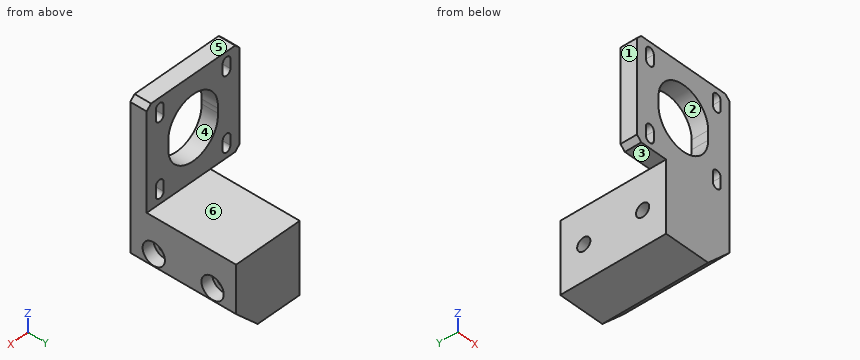
Autodesk Inventor part; units mm, degrees
ref_plane "YZ Plane" through (0, 0, 0) normal (1, 0, 0) x (0, 1, 0)
ref_plane "XZ Plane" through (0, 0, 0) normal (0, 1, 0) x (-1, 0, 0)
ref_plane "XY Plane" through (0, 0, 0) normal (0, 0, 1) x (1, 0, 0)
sketch "Sketch1" plane through (0, 0, 0) normal (0, 1, 0) x (-1, 0, 0)
  line L0 (-21.5, 21.5) -> (21.5, 21.5)
  line L1 (21.5, 21.5) -> (21.5, -21.5)
  line L2 (21.5, -21.5) -> (-21.5, -21.5)
  line L3 (-21.5, -21.5) -> (-21.5, 21.5)
  line L4 (-21.5, 21.5) -> (21.5, -21.5) construction
  line L5 (21.5, 21.5) -> (-21.5, -21.5) construction
  circle A0 centre (0, 0) radius 11.5
  circle A1 centre (15.5, 15.5) radius 1.8
  circle A2 centre (-15.5, 15.5) radius 1.8
  circle A3 centre (-15.5, -15.5) radius 1.8
  circle A4 centre (15.5, -15.5) radius 1.8
  dimension "d0" = 23
  dimension "d1" = 43
  dimension "d2" = 43
  dimension "d3" = 3.6
  dimension "d5" = 31
  dimension "d6" = 31
extrude "Extrusion1" add sketch "Sketch1" along normal blind 7
sketch "Sketch6" plane through (0, 0, 0) normal (0, -1, 0) x (1, 0, 0)
  line L0 (21.5, -21.5) -> (-21.5, -21.5)
  line L1 (-8, -21.5) -> (-8, -51.5)
  line L2 (21.5, -21.5) -> (-8, -21.5)
  line L3 (-8, -21.5) -> (-8, -51.5)
  line L4 (-8, -51.5) -> (21.5, -51.5)
  line L5 (21.5, -51.5) -> (21.5, -21.5)
  point P0 (0, 0)
  dimension "d26" = 8
  dimension "d27" = 30
extrude "Extrusion5" add sketch "Sketch6" against normal blind 45
chamfer "Chamfer1" distance 2 angle 45 3 edges at (21.5, 3.5, 21.5) (-21.5, 3.5, 21.5) (-21.5, 3.5, -21.5)
sketch "Sketch7" plane through (21.5, 0, -51.5) normal (1, 0, 0) x (0, 0, -1)
  circle A0 centre (-15, 35) radius 2.8
  circle A1 centre (-15, 10) radius 2.8
  line L0 (0, 0) -> (0, 45)
  line L1 (-71, 7) -> (-30, 7)
  line L2 (-71, 0) -> (0, 0)
  line L3 (-30, 45) -> (0, 45)
  point P0 (-51.5, 0)
  dimension "d33" = 5.6
  dimension "d34" = 5.6
  dimension "d35" = 15
  dimension "d37" = 10
  dimension "d38" = 10
extrude "Extrusion6" cut sketch "Sketch7" against normal through all
sketch "Sketch8" plane through (21.5, 0, -51.5) normal (1, 0, 0) x (0, 0, -1)
  circle A0 centre (-15, 35) radius 2.8
  circle A1 centre (-15, 35) radius 4.75
  circle A2 centre (-15, 10) radius 2.8
  circle A3 centre (-15, 10) radius 4.75
  point P0 (-51.5, 0)
  dimension "d41" = 9.5
  dimension "d42" = 9.5
extrude "Extrusion7" cut sketch "Sketch8" against normal blind 5 contours A0 | A1 | A2 | A3
chamfer "Chamfer2" distance 10 angle 45 1 edges at (21.5, 22.5, -51.5)
sketch "Sketch9" plane through (0, 0, 0) normal (0, -1, 0) x (1, 0, 0)
  line L0 (13.7, 17.5) -> (17.3, 17.5)
  line L1 (17.3, 17.5) -> (17.3, 13.5)
  line L2 (17.3, 13.5) -> (13.7, 13.5)
  line L3 (13.7, 13.5) -> (13.7, 17.5)
  circle A0 centre (15.5, 15.5) radius 1.8
  line L4 (13.7, 17.5) -> (17.3, 13.5) construction
  line L5 (17.3, 17.5) -> (13.7, 13.5) construction
  line L6 (13.7, -13.5) -> (17.3, -13.5)
  line L7 (17.3, -13.5) -> (17.3, -17.5)
  line L8 (17.3, -17.5) -> (13.7, -17.5)
  line L9 (13.7, -17.5) -> (13.7, -13.5)
  circle A1 centre (15.5, -15.5) radius 1.8
  line L10 (13.7, -13.5) -> (17.3, -17.5) construction
  line L11 (17.3, -13.5) -> (13.7, -17.5) construction
  line L12 (-17.3, 17.5) -> (-13.7, 17.5)
  line L13 (-13.7, 17.5) -> (-13.7, 13.5)
  line L14 (-13.7, 13.5) -> (-17.3, 13.5)
  line L15 (-17.3, 13.5) -> (-17.3, 17.5)
  circle A2 centre (-15.5, 15.5) radius 1.8
  line L16 (-17.3, 17.5) -> (-13.7, 13.5) construction
  line L17 (-13.7, 17.5) -> (-17.3, 13.5) construction
  line L18 (-17.3, -13.5) -> (-13.7, -13.5)
  line L19 (-13.7, -13.5) -> (-13.7, -17.5)
  line L20 (-13.7, -17.5) -> (-17.3, -17.5)
  line L21 (-17.3, -17.5) -> (-17.3, -13.5)
  circle A3 centre (-15.5, -15.5) radius 1.8
  line L22 (-17.3, -13.5) -> (-13.7, -17.5) construction
  line L23 (-13.7, -13.5) -> (-17.3, -17.5) construction
  circle A4 centre (15.5, 17.5) radius 1.8
  circle A5 centre (15.5, -17.5) radius 1.8
  circle A6 centre (15.5, -13.5) radius 1.8
  circle A7 centre (-15.5, -17.5) radius 1.8
  circle A8 centre (-15.5, -13.5) radius 1.8
  circle A9 centre (-15.5, 13.5) radius 1.8
  circle A10 centre (-15.5, 17.5) radius 1.8
  circle A11 centre (15.5, 13.5) radius 1.8
  point P0 (0, 0)
  point P1 (-17.3, 17.5)
  point P2 (13.7, 17.5)
  point P3 (17.3, 13.5)
  dimension "d48" = 4
  dimension "d49" = 4
extrude "Extrusion8" cut sketch "Sketch9" against normal blind 10
sketch "Sketch10" plane through (0, 0, 0) normal (0, -1, 0) x (1, 0, 0)
  line L0 (-11.5, 2) -> (11.5, 2)
  line L1 (11.5, 2) -> (11.5, -2)
  line L2 (11.5, -2) -> (-11.5, -2)
  line L3 (-11.5, -2) -> (-11.5, 2)
  line L4 (-11.5, 2) -> (11.5, -2) construction
  line L5 (11.5, 2) -> (-11.5, -2) construction
  circle A0 centre (0, -2) radius 11.5
  circle A1 centre (0, 2) radius 11.5
  circle A2 centre (0, 0) radius 11.5
  point P0 (11.3248, 2)
  point P1 (-11.3248, 2)
  point P2 (-11.3248, -2)
  point P3 (11.3248, -2)
  point P4 (-11.5, 0)
  point P5 (11.5, 0)
  dimension "d52" = 4
extrude "Extrusion9" cut sketch "Sketch10" against normal blind 10
sketch "Sketch4" plane through (21.5, 0, 21.5) normal (1, 0, 0) x (0, 0, -1)
  line L0 (43, 45) -> (73, 45)
  line L1 (73, 45) -> (73, 0)
  line L2 (73, 0) -> (43, 0)
  line L3 (43, 0) -> (43, 45)
  line L4 (0, 0) -> (43, 0)
  line L5 (43, 0) -> (43, 7)
  point P0 (21.5, 0)
  dimension "d17" = 30
  dimension "d18" = 45
sketch "Sketch5" plane through (21.5, 0, 21.5) normal (1, 0, 0) x (0, 0, -1)
  circle A0 centre (58, 33) radius 2.75
  circle A1 centre (58, 12) radius 2.75
  line L0 (73, 45) -> (43, 45)
  line L1 (0, 0) -> (73, 0)
  point P0 (21.5, 0)
  dimension "d21" = 12
  dimension "d22" = 12
  dimension "d23" = 5.5
properties part number "ymotorholder"
Input: part model. Units: mm. Frame: model coordinates. Face numbers are marked on the shaded views. A direction names the side the tool comes from. Give positions to 0.01 mm unless a question says otherwise; leave off trailing zeros. Order: outer loops, then holes, each group sorted by start corner. A loop starts at its lowest first (then second) coordinate and runs counter-clockwise, first axis right, second up.
1. Set-up query: the marked faces 4, 5 and 6. Return all of +Z, -Z, +X, -X, +Y, -Y with unobstructed straight access to the full face (end or side cutting, diameter ignored); none if empty.
Computed:
face 4: +Y, -Y
face 5: +Z, +X, -X, +Y, -Y
face 6: +Z, +X, -X, +Y
2. Cut plane B-B (x = -3). Return loops of the section in (y, z).
Computed:
outline: (0, -51.5) - (45, -51.5) - (45, -21.5) - (7, -21.5) - (7, -13.1) - (0, -13.1) - close; (0, 13.1) - (7, 13.1) - (7, 21.5) - (0, 21.5) - close; hole circle Ø5.6 at (10, -36.5); hole circle Ø5.6 at (35, -36.5)
3. Pin query (flat end, axial travel): pin 1 Ø9 at (x, y) = (5, 25) entering from +Z; pin 2 Ø24 at (y, z) = (27.5, -35.5) entering from -X; pin 3 Ø5.5 at (x, y) = (-13.5, 5) entering from -Z; pin 4 Ø4 at (x, z) = (-11, -2.5) entering from -Y. Return the tip coordinate at first contact, or that it passes through.
Computed:
pin 1: stops at z = -21.5
pin 2: stops at x = -8
pin 3: stops at z = -21.5
pin 4: stops at y = 0
4. Cut plane D-D (y = 10). Return loops of the section in (x, z), and give its area (3 significant figures).
Computed:
outline: (-8, -51.5) - (11.5, -51.5) - (21.5, -41.5) - (21.5, -41.25) - (16.5, -41.25) - (16.5, -39.3) - (-8, -39.3) - close; (-8, -33.7) - (16.5, -33.7) - (16.5, -31.75) - (21.5, -31.75) - (21.5, -21.5) - (-8, -21.5) - close
area: 650 mm2
5. Cut plane C-C (x = 15.5). Return loops of the section in (y, z), and give its area (3 significant figures).
Computed:
outline: (0, -47.5) - (45, -47.5) - (45, -21.5) - (7, -21.5) - (7, -19.3) - (0, -19.3) - close; (0, -11.7) - (7, -11.7) - (7, 11.7) - (0, 11.7) - close; (0, 19.3) - (7, 19.3) - (7, 21.5) - (0, 21.5) - close; hole circle Ø5.6 at (10, -36.5); hole circle Ø5.6 at (35, -36.5)
area: 1,320 mm2
6. Draft query along X for the marked faces 1, 2 and 3. Return one class per face: released by +X, released by -X, zero draft, split by the parting line, or undercut.
Computed:
face 1: released by -X
face 2: undercut
face 3: zero draft
7. Cut plane A-A (y = 4). State how many separate pieces and enclosed holes the cut face has, and give its area (3 significant figures).
Computed:
separate pieces: 1
enclosed holes: 5
area: 2,070 mm2
8. Line query: probe 1 along Y at (x, z) = (5, -36.5); probe 2 along Y at (x, z) = (18.55, -36.5); probe 3 along Z at (x, y) = (-0.5, 17). Output: solid intervals per line, ascending.
Computed:
probe 1: y = 0 to 7.2, 12.8 to 32.2, 37.8 to 45
probe 2: y = 0 to 5.25, 14.75 to 30.25, 39.75 to 45
probe 3: z = -51.5 to -21.5
